Geometry check sheet. Reference: the model listing, model coordinates, mm. A direction names the side the tool comes from. Give positions to 0.01 mm unless a question says otherwise; leave off trailing zeros. Loops run counter-clockwise (first coordinate to the right, second up) from the corner with the lowest first, then second, coordinate; pieces in that order, holes last. Notation, with made-up numbers: (27.5, 52) - (60.5, 52) arc R9 ccw to (60.5, 57) - close; hole circle Ø1 at (50.5, 35). An arc over 180 degrees is marked (long way). Use a Markdown table: item, result. Add a question column.
1. Cross-section at D-D on x = 30. Enter the section's corners in (y, z), and give its area (3 significant figures).
2. Cross-section at B-B on z = -6. Enter the section's corners in (x, y).
3. Cross-section at C-C on x = -10. Enter the section's corners in (y, z), and give its area (3 significant figures).
4. Draft check along X on faces 1 (the flat face through (35.377, -2, -1)), 2 (the flat face through (0, -2, -7.992)), 3 (the cylindrical face through (-17.4, -3.5, -0.1)), 4 (the flat face through (-34.623, -2, -1)). Enter one of: pulls with the +X half, pulls with the -X half, needs draft (parallel to the pull), parting line crosses it, or undercut.
5. Cross-section at A-A on z = 0. Enter the section's corners in (x, y).
6. Depth check by flat-ended pin: P1, Ø1.5, axis at x = 4, y = -3, coming from the +Z side; P2, Ø5, axis at x = 12.5, z = -5.5, coming from the -Y side. Enter the tip coordinate at first touch or a pass-through.
7. Set-up check for faces 5 (the flat face through (0, 0, -1)), 6 (the flat face through (0, -4.3, -5)): record each of +Z, -Z, +X, -X, +Y, -Y from which the full face is reachable in a straight line by a thin tool's end or side.
8. Material ranges on L1, parallel to Z at x = -11.5, y = -1.1; L2, parallel to Y at x = -18, z = -6; L3, parallel to Z at x = -17, y = -4.7, recorded low to high.
from build123d import *

# Parameters (mm, degrees)
F1_DEPTH       = 5
F0_W           = 70
F0_H           = 5.9
F2_DEPTH       = 4.3
F3_D           = 3
F3_CSINK_D     = 6.72
F3_CSINK_ANGLE = 90


with BuildPart() as f1:
    # F0 (on Front) → F1 (new body)
    with BuildSketch(Plane.XZ):
        Polygon((-34.6234844969, 5.539), (-34.6234844969, 0), (-34.6234844969, -2.092), (35.3765155031, -2.092), (35.3765155031, 0), (35.3765155031, 5.511366824), align=None)
    extrude(amount=F1_DEPTH)

    # F0 (on Front) → F2 (join)
    with BuildSketch(Plane.XZ):
        with Locations((0.3765155031, -5.042)):
            Rectangle(F0_W, F0_H)
    extrude(amount=F2_DEPTH)

    # F3 (through all)
    with Locations(Plane(origin=(0, 0, 0), x_dir=(1, 0, 0), z_dir=(0, 1, 0))):
        with Locations((19.6505155031, 0), (-18.8974844969, 0)):
            CounterSinkHole(F3_D / 2, F3_CSINK_D / 2, counter_sink_angle=F3_CSINK_ANGLE)


solid = f1.part
Values found:
| question | item | result |
|---|---|---|
| 1 | outline | (-5, -2.09) - (-4.3, -2.09) - (-4.3, -7.99) - (0, -7.99) - (0, 5.51) - (-5, 5.51) - close |
| 1 | area | 63.4 mm2 |
| 2 | outline | (-34.62, -4.3) - (35.38, -4.3) - (35.38, 0) - (-34.62, 0) - close |
| 3 | outline | (-5, -2.09) - (-4.3, -2.09) - (-4.3, -7.99) - (0, -7.99) - (0, 5.53) - (-5, 5.53) - close |
| 3 | area | 63.5 mm2 |
| 4 | face 1 | pulls with the +X half |
| 4 | face 2 | needs draft |
| 4 | face 3 | undercut |
| 4 | face 4 | pulls with the -X half |
| 5 | outline | (-34.62, -5) - (-20.4, -5) - (-20.4, -1.86) - (-22.26, 0) - (-34.62, 0) - close; (-17.4, -5) - (18.15, -5) - (18.15, -1.86) - (16.29, 0) - (-15.54, 0) - (-17.4, -1.86) - close; (21.15, -5) - (35.38, -5) - (35.38, 0) - (23.01, 0) - (21.15, -1.86) - close |
| 6 | P1 | stops at z = 5.52 |
| 6 | P2 | stops at y = -4.3 |
| 7 | face 5 | +Z, -Z, +X, -X, +Y |
| 7 | face 6 | -Z, +X, -X, -Y |
| 8 | L1 | z = -7.99 to 5.53 |
| 8 | L2 | y = -4.3 to 0 |
| 8 | L3 | z = -2.09 to 5.53 |
